from build123d import *

# Parameters (mm, degrees)
F0_R          = 2
F2_DEPTH      = 5
F2_DEPTH_BACK = 5
F3_DEPTH      = 14
F4_DEPTH      = 25
F4_DEPTH_BACK = 25
F5_DEPTH      = 7.6
F5_DEPTH_BACK = 7.6


with BuildPart() as f2:
    # F0 (on Front) → F2 (new body, two sides)
    with BuildSketch(Plane.XZ) as f2_sk:
        with BuildLine():
            ThreePointArc((0, 4), (1.1715728753, 1.1715728753), (4, 0))
            Line((4, 0), (29, 0))
            Line((29, 0), (29, 14))
            Line((29, 14), (4, 14))
            ThreePointArc((4, 14), (1.1715728753, 12.8284271247), (0, 10))
            Line((0, 10), (0, 4))
        make_face()
        with Locations((7, 7)):
            Circle(F0_R, mode=Mode.SUBTRACT)
        with BuildLine():
            Line((29, 14), (29, 0))
            Line((29, 0), (36, 0))
            ThreePointArc((36, 0), (34.5, 7), (36, 14))
            Line((36, 14), (29, 14))
        make_face()
    extrude(amount=-F2_DEPTH)
    extrude(f2_sk.sketch, amount=F2_DEPTH_BACK)

    # F1 (on Top) → F3 (join)
    with BuildSketch(Plane.XY):
        with BuildLine():
            Line((36, 7.6), (47, 7.6))
            Line((47, 7.6), (47, 14.6))
            Line((47, 14.6), (32, 14.6))
            ThreePointArc((32, 14.6), (29.8786796564, 13.7213203436), (29, 11.6))
            Line((29, 11.6), (29, 5))
            Line((29, 5), (36, 5))
            Line((36, 5), (36, 7.6))
        make_face()
        with BuildLine():
            ThreePointArc((29, -11.6), (29.8786796564, -13.7213203436), (32, -14.6))
            Line((32, -14.6), (47, -14.6))
            Line((47, -14.6), (47, -7.6))
            Line((47, -7.6), (36, -7.6))
            Line((36, -7.6), (36, -5))
            Line((36, -5), (29, -5))
            Line((29, -5), (29, -11.6))
        make_face()
    extrude(amount=F3_DEPTH)

    # F0 (on Front) → F4 (cut, two sides)
    with BuildSketch(Plane.XZ) as f4_sk:
        with Locations((42, 7)):
            Circle(F0_R)
        with BuildLine():
            Line((47, 14), (42, 14))
            ThreePointArc((42, 14), (45.5355339059, 12.5355339059), (47, 9))
            Line((47, 9), (47, 14))
        make_face()
        with BuildLine():
            ThreePointArc((47, 5), (45.5355339059, 1.4644660941), (42, 0))
            Line((42, 0), (47, 0))
            Line((47, 0), (47, 5))
        make_face()
    extrude(amount=-F4_DEPTH, mode=Mode.SUBTRACT)
    extrude(f4_sk.sketch, amount=F4_DEPTH_BACK, mode=Mode.SUBTRACT)

    # F0 (on Front) → F5 (cut, two sides)
    with BuildSketch(Plane.XZ) as f5_sk:
        with BuildLine():
            ThreePointArc((36, 14), (34.5, 7), (36, 0))
            Line((36, 0), (36, 14))
        make_face()
    extrude(amount=-F5_DEPTH, mode=Mode.SUBTRACT)
    extrude(f5_sk.sketch, amount=F5_DEPTH_BACK, mode=Mode.SUBTRACT)


solid = f2.part
Verification items for the finished model (mm, model axes). A direction names the side the tool comes from. Give positions to 0.01 mm unless a question says otherwise; leave off trailing zeros. Order: outer loops, then holes, each group sorted by start corner. A loop starts at its lowest first (then second) coordinate and runs counter-clockwise, first axis right, second up. Notation, with made-up numbers: (-2, -28) -> (2, -28) arc R5 cw to (2, -21) -> close; hole circle Ø6 at (40.25, -22.75). An arc over 180 degrees is marked (long way). Answer as CSV lines item,"result".
Q1. Sectioned sample at B-B on z = 7. Record the cut outline in (x, y).
Solutions:
outline,"(0, -5) -> (5, -5) -> (5, 5) -> (0, 5) -> close; (9, -5) -> (29, -5) -> (29, -11.6) arc R3 ccw to (32, -14.6) -> (40, -14.6) -> (40, -7.6) -> (34.5, -7.6) -> (34.5, 7.6) -> (40, 7.6) -> (40, 14.6) -> (32, 14.6) arc R3 ccw to (29, 11.6) -> (29, 5) -> (9, 5) -> close; (44, -14.6) -> (47, -14.6) -> (47, -7.6) -> (44, -7.6) -> close; (44, 7.6) -> (47, 7.6) -> (47, 14.6) -> (44, 14.6) -> close"
Q2. Scan lines: probe 1 along Y at (x, z) = (39, 5.5); probe 2 along X at (y, z) = (-10.25, 7); probe 3 along Z at (x, y) = (7, -0.75). Record each from-to range of solid material in increasing order.
Solutions:
probe 1,"y = -14.6 to -7.6, 7.6 to 14.6"
probe 2,"x = 29 to 40, 44 to 47"
probe 3,"z = 0 to 5, 9 to 14"
Q3. Depth check by flat-ended pin: pin 1 (3.5 mm diameter, centred on x = 7, z = 7, fed in from -Y); pin 2 (8 mm diameter, centred on y = 3, z = 7.5, fed in from +X); pin 3 (4 mm diameter, centred on x = 21, z = 5, fed in from -Y); pin 4 (7.5 mm diameter, centred on y = -9.5, z = 3.5, fed in from -X). Enter the tip coordinate at first touch or a pass-through.
Solutions:
pin 1,"passes through"
pin 2,"stops at x = 35.1"
pin 3,"stops at y = -5"
pin 4,"stops at x = 29"
Q4. Sectioned sample at C-C on y = -9.25. Record the cut outline in (x, z), plus the area to 3 significant figures.
Solutions:
outline,"(29, 0) -> (42, 0) arc R5 ccw to (47, 5) -> (47, 9) arc R5 ccw to (42, 14) -> (29, 14) -> close; hole circle Ø4 at (42, 7)"
area,"229 mm²"
Q5. Access from +Z, -Z, +X, -X, +Y, -Y to the whole of each face (thin tool, end or side, straight path). Record for faces 4 (the flat face through (29, -8, 7)), 5 (the flat face through (14, 5, 7)), 6 (the cylindrical face through (45, 11, 13)).
Solutions:
face 4,"+Z, -Z, -X, -Y"
face 5,"+Z, -Z, -X, +Y"
face 6,"+Z, +X, +Y, -Y"
Q6. Release check for a two-part mould opening along Z. For faces 1 (the cylindrical face through (34.5, 0.1, 6.9)), 2 (the flat face through (39, -14.6, 7)), 3 (the cylindrical face through (46, -11, 2)) record: +Z half, -Z half, draft (parallel to the pull), parting line (faces both ways), or undercut.
Solutions:
face 1,"undercut"
face 2,"draft"
face 3,"-Z half"
Q7. Sectioned sample at A-A on x = 39. Record the cut outline in (y, z).
Solutions:
outline,"(-14.6, 0) -> (-7.6, 0) -> (-7.6, 14) -> (-14.6, 14) -> close; (7.6, 0) -> (14.6, 0) -> (14.6, 14) -> (7.6, 14) -> close"
Q8. Sectioned sample at D-D on y = 3.75. Record the cut outline in (x, z), plus the area to 3 significant figures.
Solutions:
outline,"(0, 4) arc R4 ccw to (4, 0) -> (36, 0) arc R17.08 cw to (36, 14) -> (4, 14) arc R4 ccw to (0, 10) -> close; hole circle Ø4 at (7, 7)"
area,"470 mm²"
